from build123d import *

# Parameters (mm, degrees)
F0_R     = 8.5
F1_DEPTH = 4
F2_R     = 6
F3_DEPTH = 100
F4_R     = 1.5
F5_DEPTH = 114.9


with BuildPart() as f1:
    # F0 (on Top) → F1 (new body)
    with BuildSketch(Plane.XY):
        Circle(F0_R)
    extrude(amount=F1_DEPTH)

    # F2 (on Top) → F3 (join)
    with BuildSketch(Plane.XY):
        Circle(F2_R)
    extrude(amount=F3_DEPTH)

    # F4 (on face) → F5 (cut)
    with BuildSketch(Plane.XY.offset(100)):
        Circle(F4_R)
    extrude(amount=-F5_DEPTH, mode=Mode.SUBTRACT)


solid = f1.part
Read the model definition and answer for the solid it produces. Units are mm, in the model's axes. A direction names the side the tool comes from. Round coordinates to 2 decimals unless told otherwise and drop trailing zeros. Write each loop counter-clockwise with the first axis right and the second up, starting at its lowest first coordinate (ties: lowest second). Pieces come first, ordered by that corner, then holes. Notation, with made-up numbers: M -20,57 L 15,57 A36 ccw 15,94 Z; hole C 12,79 d2. An arc over 180 degrees is marked long. Use a Markdown table: item, result.
1) Flat-ended cylindrical pins translate along their axes: pin 1 (3 mm diameter, centred on x = -1.5, z = 48.5, fed in from +Y); pin 2 (2 mm diameter, centred on y = -6.5, z = 17, fed in from +X); pin 3 (1.5 mm diameter, centred on x = 4, z = 83, fed in from +Y); pin 4 (2 mm diameter, centred on x = 0.5, y = -4, fed in from -Z). Find the tip coordinate at first contact, or state that the pin passes through.
Answers follow:
| item | result |
|---|---|
| pin 1 | stops at y = 6 |
| pin 2 | stops at x = 2.4 |
| pin 3 | stops at y = 5.04 |
| pin 4 | stops at z = 0 |
2) The part is cut by section A-A (y = 0). Write down the section's boundary in (x, z), plus the area to 3 significant figures.
Answers follow:
| item | result |
|---|---|
| outline | M -8.5,0 L -1.5,0 L -1.5,100 L -6,100 L -6,4 L -8.5,4 Z; M 1.5,0 L 8.5,0 L 8.5,4 L 6,4 L 6,100 L 1.5,100 Z |
| area | 920 mm2 |
3) The part is cut by section D-D (y = 4.5). Write down the section's boundary in (x, z).
Answers follow:
| item | result |
|---|---|
| outline | M -7.21,0 L 7.21,0 L 7.21,4 L 3.97,4 L 3.97,100 L -3.97,100 L -3.97,4 L -7.21,4 Z |
4) Straight lines are drawn through the part: line 1 along Y through (x, z) = (0, 70); line 2 along Z through (x, y) = (-6.5, -3.75); line 3 along Y through (x, z) = (1, 84.5). For each, find the intervals that lie inside material, in ascending order. Write a range as [from, to].
Answers follow:
| item | result |
|---|---|
| line 1 | y = [-6, -1.5], [1.5, 6] |
| line 2 | z = [0, 4] |
| line 3 | y = [-5.92, -1.12], [1.12, 5.92] |
5) For a pull along Y with two mould halves and no side action, classify faces 3 (the cylindrical face through (-1.5, 0.07, 50.7)), 4 (the flat face through (1.2, -1.2, 100)), 5 (the cylindrical face through (4.57, 7.167, 1.972)) as pulls with the +Y half, pulls with the -Y half, needs draft (parallel to the pull), parting line crosses it, or undercut.
Answers follow:
| item | result |
|---|---|
| face 3 | undercut |
| face 4 | needs draft |
| face 5 | parting line crosses it |
6) A tool of negligible diameter and unlimited length cuts with its end or side. For faces 1 (the flat face through (2, 6, 4)), 2 (the flat face through (2, 0, 0)), from which of +Z, -Z, +X, -X, +Y, -Y can it reach the whole face along a straight path? Write none if from no direction.
Answers follow:
| item | result |
|---|---|
| face 1 | +Z |
| face 2 | -Z, +X, -X, +Y, -Y |
7) The part is cut by section C-C (z = 25). Write down the section's boundary in (x, y), plus the area to 3 significant figures.
Answers follow:
| item | result |
|---|---|
| outline | C 0,0 d12; hole C 0,0 d3 |
| area | 106 mm2 |
